```python
from build123d import *

# Parameters (mm, degrees)
SKETCH1_W               = 30
SKETCH1_H               = 7.8
BOSS_EXTRUDE1_DEPTH     = 3
CUT_EXTRUDE1_REACH      = 5
SKETCH2_R               = 2.25
SKETCH3_W               = 3
SKETCH3_H               = 7.8
BOSS_EXTRUDE2_DEPTH     = 75
SKETCH4_R               = 2.25
CUT_EXTRUDE2_DEPTH      = 1
CUT_EXTRUDE2_DEPTH_BACK = 31
FILLET1_R               = 3


with BuildPart() as part:
    # Sketch1 → Boss-Extrude1 (new body)
    with BuildSketch(Plane(origin=(0, 0, 0), x_dir=(1, 0, 0), z_dir=(0, 1, 0))):
        Rectangle(SKETCH1_W, SKETCH1_H)
    extrude(amount=-BOSS_EXTRUDE1_DEPTH)

    # Sketch2 → Cut-Extrude1 (cut, up to next)
    with BuildSketch(Plane(origin=(0, 0, 0), x_dir=(1, 0, 0), z_dir=(0, 1, 0)), mode=Mode.PRIVATE) as cut_extrude1_sk1:
        with Locations((-5, 0)):
            Circle(SKETCH2_R)
    cut_extrude1_tool1 = extrude(cut_extrude1_sk1.sketch, amount=-CUT_EXTRUDE1_REACH, mode=Mode.PRIVATE) & part.part
    add(cut_extrude1_tool1.solids().sort_by_distance((-5, 0, 0))[0], mode=Mode.SUBTRACT)
    # Sketch2 → Cut-Extrude1 (cut, up to next)
    with BuildSketch(Plane(origin=(0, 0, 0), x_dir=(1, 0, 0), z_dir=(0, 1, 0)), mode=Mode.PRIVATE) as cut_extrude1_sk2:
        with Locations((5, 0)):
            Circle(SKETCH2_R)
    cut_extrude1_tool2 = extrude(cut_extrude1_sk2.sketch, amount=-CUT_EXTRUDE1_REACH, mode=Mode.PRIVATE) & part.part
    add(cut_extrude1_tool2.solids().sort_by_distance((5, 0, 0))[0], mode=Mode.SUBTRACT)

    # Sketch3 → Boss-Extrude2 (add)
    with BuildSketch(Plane.XZ.offset(3)):
        with Locations((-13.5, 0)):
            Rectangle(SKETCH3_W, SKETCH3_H)
        with Locations((13.5, 0)):
            Rectangle(SKETCH3_W, SKETCH3_H)
    extrude(amount=BOSS_EXTRUDE2_DEPTH)

    # Sketch4 → Cut-Extrude2 (cut, two sides)
    with BuildSketch(Plane(origin=(15, 0, 0), x_dir=(0, 0, -1), z_dir=(1, 0, 0))) as cut_extrude2_sk:
        with Locations((0, -73.5)):
            Circle(SKETCH4_R)
    extrude(amount=CUT_EXTRUDE2_DEPTH, mode=Mode.SUBTRACT)
    extrude(cut_extrude2_sk.sketch, amount=-CUT_EXTRUDE2_DEPTH_BACK, mode=Mode.SUBTRACT)

    # Fillet1
    fillet1_edges = [part.edges().sort_by_distance(p)[0] for p in [
        (-13.5, -78, -3.9),
        (-13.5, -78, 3.9),
        (13.5, -78, 3.9),
        (13.5, -78, -3.9),
    ]]
    fillet(fillet1_edges, radius=FILLET1_R)


solid = part.part
```
For this review, take the finished solid that the model builds, in its own axes (mm). A direction names the side the tool comes from. Coordinates: 2 decimals unless noted, no trailing zeros. Order: outer loops, then holes, each group sorted by start corner. A loop starts at its lowest first (then second) coordinate and runs counter-clockwise, first axis right, second up. Notation, with made-up numbers: (49.5, 66) -> (65.5, 66) arc R13 ccw to (65.5, 81) -> close; hole circle Ø4 at (37, 43). An arc over 180 degrees is marked (long way). Use CSV: the item, a comma, the result in double quotes. Start each with the question number.
Item 1: Insertion check: pin 1 (2.5 mm diameter, centred on x = -2, z = 0, fed in from -Y). The pin has a flat end and moves straight along its axis. Give the tip position at first contact, or say it passes through.
Item 2: We need section D-D, the plane x = 5. Give the boundary of the cut face in (y, z), then the cut area to 3 significant figures.
Item 3: Wall thickness on probe 1 along X at (y, z) = (-0.65, 0); probe 2 along X at (y, z) = (-41, 2.5); probe 3 along Z at (x, y) = (-5, -1.4): over which ranges is each line inside the solid? List them lowest first.
Item 4: We need section B-B, the plane y = -6. Give the boundary of the cut face in (x, z).
Item 5: Draft analysis for pull direction Y (two halves, no side actions). For faces 3 (the face through (-13.479, -75.696, 0.488)), 4 (the face through (0, 0, 0)), 5 (the face through (-12.3, -31.8, 3.9)), 6 (the face through (13.52, -77.1, -3.04)), state which applies: pulls with the +Y half, pulls with the -Y half, needs draft (parallel to the pull), parting line crosses it, or undercut.
Item 6: For faces 1 (the face through (-12, -40, 0)), 2 (the face through (-14, -78, 0)), list the 3-axis set-ups (+Z, -Z, +X, -X, +Y, -Y) from which the entire face can be reached by the end or side of a thin tool; tool diameter is ignored.
Item 7: We need section A-A, the plane z = 0. Give the boundary of the cut face in (x, y).
Item 8: We need section C-C, the plane y = -73.5. Give the boundary of the cut face in (x, z).
Derived:
1,pin 1,"stops at y = -3"
2,outline,"(-3, -3.9) -> (0, -3.9) -> (0, -2.25) -> (-3, -2.25) -> close; (-3, 2.25) -> (0, 2.25) -> (0, 3.9) -> (-3, 3.9) -> close"
2,area,"9.90 mm^2"
3,probe 1,"x = -15 to -7.25, -2.75 to 2.75, 7.25 to 15"
3,probe 2,"x = -15 to -12, 12 to 15"
3,probe 3,"z = -3.9 to -2.25, 2.25 to 3.9"
4,outline,"(-15, -3.9) -> (-12, -3.9) -> (-12, 3.9) -> (-15, 3.9) -> close; (12, -3.9) -> (15, -3.9) -> (15, 3.9) -> (12, 3.9) -> close"
5,face 3,"undercut"
5,face 4,"pulls with the +Y half"
5,face 5,"needs draft"
5,face 6,"pulls with the -Y half"
6,face 1,"+Z, -Z, -Y"
6,face 2,"+Z, -Z, +X, -X, -Y"
7,outline,"(-15, -78) -> (-12, -78) -> (-12, -75.75) -> (-15, -75.75) -> close; (-15, -71.25) -> (-12, -71.25) -> (-12, -3) -> (-7.25, -3) -> (-7.25, 0) -> (-15, 0) -> close; (-2.75, -3) -> (2.75, -3) -> (2.75, 0) -> (-2.75, 0) -> close; (7.25, -3) -> (12, -3) -> (12, -71.25) -> (15, -71.25) -> (15, 0) -> (7.25, 0) -> close; (12, -78) -> (15, -78) -> (15, -75.75) -> (12, -75.75) -> close"
8,outline,"(-15, -3.9) -> (-12, -3.9) -> (-12, -2.25) -> (-15, -2.25) -> close; (-15, 2.25) -> (-12, 2.25) -> (-12, 3.9) -> (-15, 3.9) -> close; (12, -3.9) -> (15, -3.9) -> (15, -2.25) -> (12, -2.25) -> close; (12, 2.25) -> (15, 2.25) -> (15, 3.9) -> (12, 3.9) -> close"
